Autodesk Inventor part; units mm, degrees
ref_plane "YZ Plane" through (0, 0, 0) normal (1, 0, 0) x (0, 1, 0)
ref_plane "XZ Plane" through (0, 0, 0) normal (0, 1, 0) x (-1, 0, 0)
ref_plane "XY Plane" through (0, 0, 0) normal (0, 0, 1) x (1, 0, 0)
sketch "Sketch1" plane through (0, 0, 0) normal (0, 0, 1) x (1, 0, 0)
  circle A0 centre (0.0338, 1.5) radius 28.5
  arc A1 (-1.1621, 26.972) -> (1.1984, 26.9734) centre (0.0338, 1.5) ccw
  line L0 (-1.1621, 26.972) -> (0.0338, 1.5)
  line L1 (0.0338, 1.5) -> (1.1984, 26.9734)
  arc A2 (1.3007, 29.9718) -> (-1.3028, 29.9687) centre (0.0338, 1.5) ccw
  circle A3 centre (1.3379, 26.9666) radius 2.5
  point P0 (1.3508, 29.9696)
  dimension "d53" = 5
  dimension "d22" = 57
  dimension "d23" = 51
sketch "Sketch2" plane through (0, 0, 0) normal (0, 0, 1) x (1, 0, 0)
  circle A0 centre (0, 0) radius 28.5
  circle A1 centre (0, 0) radius 10
  circle A2 centre (0, 0) radius 31.5
  dimension "d10" = 57
  dimension "d32" = 63
  dimension "d37" = 20
extrude "Extrusion5" add sketch "Sketch2" along normal blind 31 contours A0
extrude "Extrusion9" add sketch "Sketch2" against normal blind 9 contours A0 | A2
sketch "Sketch3" plane through (0, 0, 31) normal (0, 0, 1) x (1, 0, 0)
  circle A0 centre (0, 0) radius 31.5
  circle A1 centre (0, 0) radius 10
  dimension "d38" = 63
  dimension "d40" = 20
extrude "Extrusion11" add sketch "Sketch3" along normal blind 4
extrude "Extrusion15" cut sketch "Sketch1" along normal through all both and the other way through all contours A3 A1 L1 | A3 L1 A1
pattern_circular "Circular Pattern4" count 18 over 360 about axis through (0, 0, 0) along (0, 0, 1) of "Extrusion15"
sketch "Sketch7" plane through (0, 0, -9) normal (0, 0, -1) x (-1, 0, 0)
  circle A0 centre (0, 0) radius 10
  circle A1 centre (0, 0) radius 31.5
  circle A2 centre (0, 0) radius 14
  dimension "d62" = 28
extrude "Extrusion17" cut sketch "Sketch7" against normal blind 27 contours A2
sketch "Sketch8" plane through (0, 0, 35) normal (0, 0, 1) x (1, 0, 0)
  circle A0 centre (0, 0) radius 14
  dimension "d65" = 28
extrude "Extrusion18" cut sketch "Sketch8" against normal blind 8
ref_plane "Work Plane2" through (0, 0, 15.5) normal (0, 0, 1) x (1, 0, 0)
equation "\"d53\" = 2 * SzíjFogakSugaraA"
equation "\"d22\" = 0.5 * NagyKerekAtmero"
equation "\"d23\" = 0.5 * NagyKerekAtmero - 2 * SzíjSugarKözépontEltolásaAzAlaptolA"
equation "\"d10\" = 0.5 * NagyKerekAtmero"
equation "\"d32\" = 0.5 * NagyKerekAtmero + 2 * NagyKerekPeremMagasaga"
equation "\"d37\" = NgyKerekFurat"
equation "\"d15\" = SzíjSzélességB"
equation "\"d38\" = 0.5 * NagyKerekAtmero + 2 * NagyKerekPeremMagasaga"
equation "\"d40\" = NgyKerekFurat"
equation "\"d54\" = NagyKerekPeremSzélesege"
equation "\"d63\" = NagyKerekPeremSzélesege + 0.5 * SzíjSzélességB + 0.5 * KisKerekCSapagySzeleseg"
equation "\"SzíjSzélességA\" = 31"
equation "\"SzíjAlapVastagságA\" = 3"
equation "\"SzíjFogakSugaraA\" = 2.5"
equation "\"SzíjSugarKözépontEltolásaAzAlaptolA\" = 3"
equation "\"NagyKerekAtmero\" = 114"
equation "\"SzíjSzélességB\" = 31"
equation "\"SzíjFogakSugaraB\" = 2.5"
equation "\"SzíjSugarKözépontEltolásaAzAlaptolB\" = 3"
equation "\"SzíjAlapVastagságB\" = 3"
equation "\"NagyKerekPeremSzélesege\" = 4"
equation "\"NagyKerekPeremMagasaga\" = 3"
equation "\"NgyKerekFurat\" = 20"
equation "\"NagyKerekTengelyVastagsag\" = 14"
equation "\"NagyKerékCsapágySzéleseg\" = 15"
equation "\"NagyKerekTengelyVastagság\" = 14"
equation "\"NagyKerékCsapágyBelsőÁtmérő\" = 12"
equation "\"TartoCsőFalVastagsága\" = 2"
equation "\"KisCsoBelsoFalvastagsag\" = 2"
equation "\"OrsoTengelyAtmeroje\" = 8"
equation "\"KisCsaoagyKulsoAtmero\" = 18"
equation "\"CsigaHajtásFogasKerékÁtmérő\" = 56"
equation "\"ZártSzelvényFalVastagság\" = 2"
equation "\"NagyFogaskerekSzelesege\" = 8"
equation "\"LemezVastagsag\" = 2"
equation "\"ZártSzelvényBelsőÁtmérő\" = 12"
equation "\"ForgoTalpKarBeugrasztas\" = 82"
equation "\"KisKerekCSapagySzeleseg\" = 15"
equation "\"NagyKerékSzélesege\" = 75"
properties part number "NagyKerek" material "Nylon, molybdenum disulphide"
Geometry check sheet. Reference: the model listing, model coordinates, mm. A direction names the side the tool comes from. Give positions to 0.01 mm unless a question says otherwise; leave off trailing zeros. Order: outer loops, then holes, each group sorted by start corner. A loop starts at its lowest first (then second) coordinate and runs counter-clockwise, first axis right, second up. Notation, with made-up numbers: (-16, 89.5) - (30, 89.5) arc R17 ccw to (30, 112.5) - close; hole circle Ø10 at (-28, 11.5). An arc over 180 degrees is marked (long way). Write item = value, one per line. Start each with the question number.
1) Section check B-B (y = 0). Enter the section's corners in (x, z).
2) Draft check along Y on faces 1 (the cylindrical face through (24.29, 3.48, 13.31)), 2 (the cylindrical face through (6.294, 27.796, 15.283)), 3 (the cylindrical face through (-4.101, 31.232, -4.437)). Enter one of: released by +Y, released by -Y, zero draft, split by the parting line, or undercut.
3) Scan lines: L1, parallel to Y at x = -18, z = -1; L2, parallel to Z at x = 9.5, y = 27.5; L3, parallel to X at y = 12, z = 31.5. Record each from-to range of solid material in increasing order.
4) Access from +Z, -Z, +X, -X, +Y, -Y to the whole of each face (thin tool, end or side, straight path). Record for faces 4 (the cylindrical face through (-20.925, 19.349, 15.283)), 5 (the cylindrical face through (-12.932, -5.362, 4.311)), 6 (the cylindrical face through (12.932, -5.362, 31.056)), 7 (the cylindrical face through (-6.294, -27.796, 15.283)), 8 (the flat face through (28, 7, 31)).
5) Gauge pin test, flat ends, axial feed: pin 1 Ø1.5 at (x, z) = (4, 24) entering from +Y; pin 2 Ø2 at (x, z) = (-22, 10.5) entering from -Y; pin 3 Ø4 at (x, z) = (-23, 17.5) entering from +Y. Record the tip position at first contact, or that the pin passes through.
6) Section check A-A (y = 7). Enter the section's corners in (x, z).
Geometry check:
q1.outline = (-31.5, -9) - (-14, -9) - (-14, 18) - (-10, 18) - (-10, 27) - (-14, 27) - (-14, 35) - (-31.5, 35) - (-31.5, 31) - (-28.5, 31) - (-28.5, 0) - (-31.5, 0) - close; (10, 18) - (14, 18) - (14, -9) - (31.5, -9) - (31.5, 0) - (28.5, 0) - (28.5, 31) - (31.5, 31) - (31.5, 35) - (14, 35) - (14, 27) - (10, 27) - close
q2.face_1 = undercut
q2.face_2 = released by +Y
q2.face_3 = split by the parting line
q3.L1 = -25.85 to -22.27, -17.32 to 19.68, 23.36 to 25.85
q3.L2 = -9 to 0, 31 to 35
q3.L3 = -29.12 to -7.21, 7.21 to 21.54, 26.5 to 29.12
q4.face_4 = -X, +Y
q4.face_5 = -Z
q4.face_6 = +Z
q4.face_7 = -X, -Y
q4.face_8 = none
q5.pin_1 = 28.29
q5.pin_2 = -19.27
q5.pin_3 = 19.27
q6.outline = (-30.71, -9) - (-28.62, -9) - (-28.62, 0) - (-30.71, 0) - close; (-30.71, 31) - (-28.62, 31) - (-28.62, 35) - (-30.71, 35) - close; (-24.03, -9) - (-12.12, -9) - (-12.12, 18) - (-7.14, 18) - (-7.14, 27) - (-12.12, 27) - (-12.12, 35) - (-24.03, 35) - close; (7.14, 18) - (12.12, 18) - (12.12, -9) - (30.71, -9) - (30.71, 0) - (27.63, 0) - (27.63, 31) - (30.71, 31) - (30.71, 35) - (12.12, 35) - (12.12, 27) - (7.14, 27) - close
